from build123d import *

# Parameters (mm, degrees)
SKETCH1_W          = 38.1
SKETCH1_H          = 38.1
SKETCH1_R          = 13.183
EXTRUDE1_DEPTH     = 9.4996
CUT_EXTRUDE1_DEPTH = 5.5118
HOLE1_D            = 5.7912
HOLE1_DEPTH        = 3.9878


with BuildPart() as part:
    # Sketch1 → Extrude1 (new body)
    with BuildSketch(Plane.XY):
        Rectangle(SKETCH1_W, SKETCH1_H)
        Circle(SKETCH1_R, mode=Mode.SUBTRACT)
    extrude(amount=-EXTRUDE1_DEPTH)

    # Sketch2 → Cut-Extrude1 (cut)
    with BuildSketch(Plane(origin=(0, 0, -9.4996), x_dir=(1, 0, 0), z_dir=(0, 0, -1))):
        with BuildLine():
            Line((19.05, 19.05), (19.05, 7.324620334))
            ThreePointArc((19.05, 7.324620334), (11.009543879, 11.009543879), (7.324620334, 19.05))
            Line((7.324620334, 19.05), (19.05, 19.05))
        make_face()
        with BuildLine():
            Line((19.05, -19.05), (19.05, -7.324620334))
            ThreePointArc((19.05, -7.324620334), (11.009543879, -11.009543879), (7.324620334, -19.05))
            Line((7.324620334, -19.05), (19.05, -19.05))
        make_face()
        with BuildLine():
            Line((-19.05, -19.05), (-7.324620334, -19.05))
            ThreePointArc((-7.324620334, -19.05), (-11.009543879, -11.009543879), (-19.05, -7.324620334))
            Line((-19.05, -7.324620334), (-19.05, -19.05))
        make_face()
        with BuildLine():
            Line((-19.05, 19.05), (-7.324620334, 19.05))
            ThreePointArc((-7.324620334, 19.05), (-11.009543879, 11.009543879), (-19.05, 7.324620334))
            Line((-19.05, 7.324620334), (-19.05, 19.05))
        make_face()
    extrude(amount=-CUT_EXTRUDE1_DEPTH, mode=Mode.SUBTRACT)

    # Hole1
    with Locations(Plane(origin=(0, 0, -3.9878), x_dir=(-1, 0, 0), z_dir=(0, 0, -1))):
        with Locations((14.5034, 14.5034), (14.5034, -14.5034), (-14.5034, 14.5034), (-14.5034, -14.5034)):
            Hole(HOLE1_D / 2, depth=HOLE1_DEPTH)

    # Sketch5 → Cut-Revolve1 (revolve, cut)
    with BuildSketch(Plane(origin=(0, 0, 0), x_dir=(0, 0, -1), z_dir=(1, 0, 0)), mode=Mode.PRIVATE) as cut_revolve1_sk:
        Polygon((9.4996, 13.183), (9.4996, 14.351), (8.3316, 13.183), align=None)
        Polygon((1.168, 13.183), (0, 13.183), (0, 14.351), align=None)
    revolve(cut_revolve1_sk.sketch.rotate(Axis((0, 0, 7.380919067), (0, 0, -1)), 90), axis=Axis((0, 0, 7.380919067), (0, 0, -1)), mode=Mode.SUBTRACT)  # turned: the seam where the file's is

    # Sketch6 → Cut-Revolve2 (revolve, cut)
    with BuildSketch(Plane(origin=(0, 0, 0), x_dir=(1, 0, 0), z_dir=(0, 1, 0))):
        Polygon((15.875, 9.4996), (16.256, 9.1186), (16.637, 9.4996), align=None)
    revolve(axis=Axis((0, 0, 0), (0, 0, -1)), mode=Mode.SUBTRACT)


solid = part.part
Could you check a few things on this model? Use its own coordinates, in mm. A direction names the side the tool comes from. Coordinates: 2 decimals unless noted, no trailing zeros. Order: outer loops, then holes, each group sorted by start corner. A loop starts at its lowest first (then second) coordinate and runs counter-clockwise, first axis right, second up. Notation, with made-up numbers: (23.25, -38.75) - (38.25, -38.75) arc R9 cw to (38.25, -28.75) - close; hole circle Ø7 at (-38, 19). An arc over 180 degrees is marked (long way). Answer in a Markdown table with one row per item. Add a question column.
(1) If we section it at A-A, the plane x = 0: Please give me the cut outline in (y, z) (3 decimals).
(2) Will these pins go through, and if not, where does the flat tip stop? pin 1 (3.5 mm diameter, centred on x = -14.5, y = -14.5, fed in from +Z); pin 2 (7.5 mm diameter, centred on x = 14.5, y = -14.5, fed in from -Z).
(3) If we section it at B-B, the plane z = -6.5: Please give me the cut outline in (x, y).
(4) If we mould it in two halves opening along Y, with no side actions, what happens to faces 5 (the face through (-10.92, -11.1, -6.78)), 6 (the face through (16.364, 0.136, -9.227)), 7 (the face through (-12, -12, -3.988))? For each: released by +Y, released by -Y, zero draft, split by the parting line, or undercut.
(5) On a 3-axis mill with a long thin cutter (end or side, diameter ignored), from which of +Z, -Z, +X, -X, +Y, -Y can I reach the whole of each face in a straight line? I mean faces 1 (the face through (-12, 12, -3.988)), 2 (the face through (0.136, -16.364, -9.227)), 3 (the face through (12, -12, -3.988)), 4 (the face through (13.1, 11.8, -3.988)). Say none if no direction works.
(6) If we section it at D-D, the plane z = -3.5: Please give me the cut outline in (x, y).
(7) I need wall thicknesses on L1, parallel to Y at x = 16, z = -2.75; L2, parallel to Z at x = -12, y = 17.5; L3, parallel to X at y = 11.5, z = -8.5. Which ranges of each line are inside material? Lowest first, please.
Results are:
| question | item | result |
|---|---|---|
| 1 | outline | (-19.05, -9.5) - (-16.637, -9.5) - (-16.256, -9.119) - (-15.875, -9.5) - (-14.351, -9.5) - (-13.183, -8.332) - (-13.183, -1.168) - (-14.351, 0) - (-19.05, 0) - close; (13.183, -8.332) - (14.351, -9.5) - (15.875, -9.5) - (16.256, -9.119) - (16.637, -9.5) - (19.05, -9.5) - (19.05, 0) - (14.351, 0) - (13.183, -1.168) - close |
| 2 | pin 1 | passes through |
| 2 | pin 2 | stops at z = -3.99 |
| 3 | outline | (-19.05, -7.32) arc R12.7 cw to (-7.32, -19.05) - (7.32, -19.05) arc R12.7 cw to (19.05, -7.32) - (19.05, 7.32) arc R12.7 cw to (7.32, 19.05) - (-7.32, 19.05) arc R12.7 cw to (-19.05, 7.32) - close; hole circle Ø26.37 at (0, 0) |
| 4 | face 5 | released by -Y |
| 4 | face 6 | undercut |
| 4 | face 7 | zero draft |
| 5 | face 1 | -Z, -X, +Y |
| 5 | face 2 | -Z |
| 5 | face 3 | -Z, +X, -Y |
| 5 | face 4 | -Z, +X, +Y |
| 6 | outline | (-19.05, -19.05) - (19.05, -19.05) - (19.05, 19.05) - (-19.05, 19.05) - close; hole circle Ø5.79 at (-14.5, -14.5); hole circle Ø5.79 at (-14.5, 14.5); hole circle Ø26.37 at (0, 0); hole circle Ø5.79 at (14.5, -14.5); hole circle Ø5.79 at (14.5, 14.5) |
| 7 | L1 | y = -19.05 to -16.98, -12.02 to 12.02, 16.98 to 19.05 |
| 7 | L2 | z = -3.99 to 0 |
| 7 | L3 | x = -10.54 to -6.78, 6.78 to 10.54 |
